Here's how the part is built. I have some questions about the finished solid (model axes, mm). Face numbers are marked on the shaded views. A direction names the side the tool comes from. Coordinates: 2 decimals unless noted, no trailing zeros. Write each loop counter-clockwise with the first axis right and the second up, starting at its lowest first coordinate (ties: lowest second). Pieces come first, ordered by that corner, then holes. Notation, with made-up numbers: M 68.25,-23 L 104.25,-23 A17 cw 104.25,-19 Z; hole C -31,54.5 d8. An arc over 180 degrees is marked long. Use a Markdown table: item, result.
```python
from build123d import *

# Parameters (mm, degrees)
CROQUIS1_R                 = 35.5
CROQUIS1_R_2               = 3.25
SALIENTE_EXTRUIR1_DEPTH    = 5
CROQUIS9_R                 = 19.85
CROQUIS9_R_2               = 3.25
SALIENTE_EXTRUIR4_DEPTH    = 35
CORTAR_EXTRUIR4_DEPTH      = 36.5
CORTAR_EXTRUIR4_DEPTH_BACK = 36.5
CROQUIS11_R                = 35.5
CROQUIS11_R_2              = 3.25
SALIENTE_EXTRUIR5_DEPTH    = 7.5
CROQUIS13_R                = 5
CORTAR_EXTRUIR5_DEPTH      = 7.5
CORTAR_EXTRUIR7_DEPTH      = 13.5


with BuildPart() as part:
    # Croquis1 → Saliente-Extruir1 (new body)
    with BuildSketch(Plane.XY):
        Circle(CROQUIS1_R)
        with Locations((17.67766953, 17.67766953)):
            Circle(CROQUIS1_R_2, mode=Mode.SUBTRACT)
        with Locations((17.67766953, -17.67766953)):
            Circle(CROQUIS1_R_2, mode=Mode.SUBTRACT)
        with Locations((-17.67766953, -17.67766953)):
            Circle(CROQUIS1_R_2, mode=Mode.SUBTRACT)
        with Locations((-17.67766953, 17.67766953)):
            Circle(CROQUIS1_R_2, mode=Mode.SUBTRACT)
        Circle(CROQUIS1_R_2, mode=Mode.SUBTRACT)
    extrude(amount=SALIENTE_EXTRUIR1_DEPTH)

    # Croquis9 → Saliente-Extruir4 (add)
    with BuildSketch(Plane.XY.offset(5)):
        Circle(CROQUIS9_R)
        Circle(CROQUIS9_R_2, mode=Mode.SUBTRACT)
    extrude(amount=SALIENTE_EXTRUIR4_DEPTH)

    # Croquis10 → Cortar-Extruir4 (cut, two sides)
    with BuildSketch(Plane(origin=(0, 0, 0), x_dir=(1, 0, 0), z_dir=(0, 1, 0))) as cortar_extruir4_sk:
        with BuildLine():
            Line((0, -29), (0, -40))
            Line((0, -40), (-6, -40))
            Line((-6, -40), (-6, -23))
            ThreePointArc((-6, -23), (4.242640687, -18.757359313), (0, -29))
        make_face()
    extrude(amount=CORTAR_EXTRUIR4_DEPTH, mode=Mode.SUBTRACT)
    extrude(cortar_extruir4_sk.sketch, amount=-CORTAR_EXTRUIR4_DEPTH_BACK, mode=Mode.SUBTRACT)

    # Croquis11 → Saliente-Extruir5 (add)
    with BuildSketch(Plane(origin=(0, 0, 0), x_dir=(-1, 0, 0), z_dir=(0, 0, -1))):
        Circle(CROQUIS11_R)
        with Locations((17.67766953, -17.67766953)):
            Circle(CROQUIS11_R_2, mode=Mode.SUBTRACT)
        Circle(CROQUIS11_R_2, mode=Mode.SUBTRACT)
        with Locations((-17.67766953, -17.67766953)):
            Circle(CROQUIS11_R_2, mode=Mode.SUBTRACT)
        with Locations((17.67766953, 17.67766953)):
            Circle(CROQUIS11_R_2, mode=Mode.SUBTRACT)
        with Locations((-17.67766953, 17.67766953)):
            Circle(CROQUIS11_R_2, mode=Mode.SUBTRACT)
    extrude(amount=SALIENTE_EXTRUIR5_DEPTH)

    # Croquis13 → Cortar-Extruir5 (cut)
    with BuildSketch(Plane.XY.offset(5)):
        with Locations((-17.67766953, 17.67766953)):
            Circle(CROQUIS13_R)
        with Locations((17.67766953, 17.67766953)):
            Circle(CROQUIS13_R)
        with Locations((17.67766953, -17.67766953)):
            Circle(CROQUIS13_R)
        with Locations((-17.67766953, -17.67766953)):
            Circle(CROQUIS13_R)
        with BuildLine():
            Line((-20, -29.330018752), (20, -29.330018752))
            ThreePointArc((20, -29.330018752), (0, -35.5), (-20, -29.330018752))
        make_face()
    extrude(amount=-CORTAR_EXTRUIR5_DEPTH, mode=Mode.SUBTRACT)

    # Croquis15 → Cortar-Extruir7 (cut, through all)
    with BuildSketch(Plane.XY.offset(5)):
        with BuildLine():
            Line((20, -29.330018752), (-20, -29.330018752))
            ThreePointArc((-20, -29.330018752), (0, -35.5), (20, -29.330018752))
        make_face()
    extrude(amount=-CORTAR_EXTRUIR7_DEPTH, mode=Mode.SUBTRACT)


solid = part.part
```
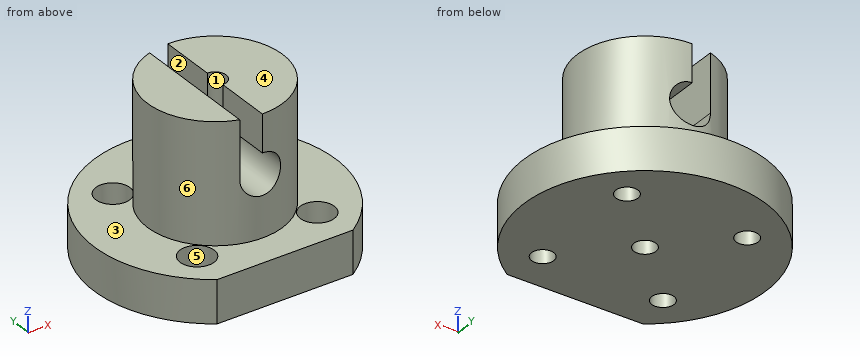
1. We'd pull the mould along X, two halves only. Please class the marked faces 4, 5 and 6: +X half, -X half, draft (parallel to the pull), parting line (faces both ways), or undercut.
Answers follow:
| item | result |
|---|---|
| face 4 | draft |
| face 5 | undercut |
| face 6 | parting line |
2. Which directions (+Z, -Z, +X, -X, +Y, -Y) give clear straight access to the entire face, cutting with the end or side of a thin tool? Please do the marked faces 1, 2 and 3.
Answers follow:
| item | result |
|---|---|
| face 1 | +Z, -Z |
| face 2 | +Z, +Y, -Y |
| face 3 | +Z |
3. Suppose I cut it at D-D on z = -4. Write out the boundary of the cut face in (x, y).
Answers follow:
| item | result |
|---|---|
| outline | M -20,-29.33 L 20,-29.33 A35.5 ccw long Z; hole C -17.68,-17.68 d6.5; hole C -17.68,17.68 d6.5; hole C 0,0 d6.5; hole C 17.68,-17.68 d6.5; hole C 17.68,17.68 d6.5 |
4. Suppose I cut it at A-A on z = 31.5. Write out the boundary of the cut face in (x, y).
Answers follow:
| item | result |
|---|---|
| outline | M -6,-18.92 L -6,18.92 A19.85 ccw Z; M 0,-19.85 A19.85 ccw 0,19.85 L 0,3.25 A3.25 cw 0,-3.25 Z |
5. Suppose I cut it at B-B on y = 0. Write out the boundary of the cut face in (x, z).
Answers follow:
| item | result |
|---|---|
| outline | M -35.5,-7.5 L -3.25,-7.5 L -3.25,17.96 A6 cw -6,23 L -6,40 L -19.85,40 L -19.85,5 L -35.5,5 Z; M 3.25,-7.5 L 35.5,-7.5 L 35.5,5 L 19.85,5 L 19.85,40 L 3.25,40 L 3.25,28.04 A6 cw 3.25,17.96 Z |
6. Will these pins go through, and if not, where does the flat tip stop? pin 1 Ø8 at (x, z) = (-18.5, 5) entering from +Y; pin 2 Ø8 at (x, y) = (-10, 24.5) entering from +Z; pin 3 Ø12 at (y, z) = (-14.5, 33) entering from -X.
Answers follow:
| item | result |
|---|---|
| pin 1 | stops at y = 32.4 |
| pin 2 | stops at z = 5 |
| pin 3 | stops at x = -17.94 |
7. Suppose I cut it at C-C on y = 16.5. Write out the boundary of the cut face in (x, z), and give its area (3 significant figures).
Answers follow:
| item | result |
|---|---|
| outline | M -31.43,-7.5 L -20.71,-7.5 L -20.71,-2.5 L -22.54,-2.5 L -22.54,5 L -31.43,5 Z; M -14.65,-7.5 L 14.65,-7.5 L 14.65,-2.5 L 12.82,-2.5 L 12.82,5 L 11.04,5 L 11.04,40 L 0,40 L 0,29 A6 cw long -6,23 L -6,40 L -11.04,40 L -11.04,5 L -12.82,5 L -12.82,-2.5 L -14.65,-2.5 Z; M 20.71,-7.5 L 31.43,-7.5 L 31.43,5 L 22.54,5 L 22.54,-2.5 L 20.71,-2.5 Z |
| area | 1,170 mm2 |
8. I need wall thicknesses on probe 1 along Y at (x, z) = (0, -6); probe 2 along Z at (x, y) = (18.5, 7.5); probe 3 along X at (y, z) = (21, -1.5). Which ranges of each line are inside material? Lowest first, please.
Answers follow:
| item | result |
|---|---|
| probe 1 | y = -29.33 to -3.25, 3.25 to 35.5 |
| probe 2 | z = -7.5 to 5 |
| probe 3 | x = -28.62 to -21.41, -13.94 to 13.94, 21.41 to 28.62 |
